Could you check a few things on this model? Use its own coordinates, in mm. A direction names the side the tool comes from. Give positions to 0.01 mm unless a question says otherwise; leave off trailing zeros. Loops run counter-clockwise (first coordinate to the right, second up) from the corner with the lowest first, then second, coordinate; pieces in that order, holes last. Notation, with made-up numbers: (70.25, 31.5) - (115.25, 31.5) arc R21 ccw to (115.25, 57.5) - close; hole circle Ø8 at (5.5, 80.5). An arc over 180 degrees is marked (long way). Write each question's results on one line, items separated by ' | '. Start each with the question number.
(1) Suppose I cut it at A-A (z = 18.5). Please give me the cut outline in (x, y), and give its area (3 significant figures).
(2) Suppose I cut it at D-D (z = -1). Please give me the cut outline in (x, y).
(3) If we mould it in two halves opening along X, with no side actions, what happens to faces 6 (the face through (11.5, 14, -13)), 7 (the face through (0, 0, 0)), 8 (the face through (0, 1.5, 0))? For each: released by +X, released by -X, zero draft, split by the parting line, or undercut.
(4) On a 3-axis mill with a long thin cutter (end or side, diameter ignored), from which of +Z, -Z, +X, -X, +Y, -Y can I reach the whole of each face in a straight line? I mean faces 1 (the face through (2.5, 13.8, -20.5)), 2 (the face through (2, 14, -9)), 3 (the face through (-11, 14, -5.5)), 4 (the face through (-4, 14, -13.5)), 5 (the face through (-11.5, 14, -13)). Say none if no direction works.
(5) Suppose I cut it at C-C (x = -8.5). Please give me the cut outline in (y, z).
(6) For pin 1 (2 mm diameter, centred on y = 19.5, z = -18.5, fed in from -X); pin 2 (1.1 mm diameter, centred on x = 2.5, y = 17, fed in from +Z); pin 3 (7.5 mm diameter, centred on y = 13, z = -7.5, fed in from +X), each with a flat end and sliding along its axis, tell me the tip position at first contact or that it passes through.
(7) Suppose I cut it at B-B (x = -18.5). Please give me the cut outline in (y, z).
(8) I need wall thicknesses on line 1 (Z direction, x = 18.5, y = 0.6); line 2 (X direction, y = 22, z = -12). Which ranges of each line are inside material? Lowest first, please.
from build123d import *

# Parameters (mm, degrees)
SKETCH1_W           = 43
SKETCH1_H           = 43
BOSS_EXTRUDE1_DEPTH = 1.5
SKETCH2_R           = 1.5
CUT_EXTRUDE1_DEPTH  = 2.5
BOSS_EXTRUDE2_DEPTH = 25


with BuildPart() as part:
    # Sketch1 → Boss-Extrude1 (new body)
    with BuildSketch(Plane(origin=(0, 0, 0), x_dir=(1, 0, 0), z_dir=(0, 1, 0))):
        Rectangle(SKETCH1_W, SKETCH1_H)
    extrude(amount=BOSS_EXTRUDE1_DEPTH)

    # Sketch2 → Cut-Extrude1 (cut, through all)
    with BuildSketch(Plane(origin=(0, 1.5, 0), x_dir=(1, 0, 0), z_dir=(0, 1, 0))):
        with Locations((-18.5, 18.5)):
            Circle(SKETCH2_R)
        with Locations((18.5, 18.5)):
            Circle(SKETCH2_R)
        with Locations((18.5, -18.5)):
            Circle(SKETCH2_R)
        with Locations((-18.5, -18.5)):
            Circle(SKETCH2_R)
    extrude(amount=-CUT_EXTRUDE1_DEPTH, mode=Mode.SUBTRACT)

    # Sketch3 → Boss-Extrude2 (add)
    with BuildSketch(Plane(origin=(0, 1.5, 0), x_dir=(1, 0, 0), z_dir=(0, 1, 0))):
        Polygon((-7, 5.5), (-7, 12.5), (-10.5, 12.5), (-10.5, 5.5), (-11.5, 5.5), (-11.5, 20.5), (-10.5, 20.5), (-10.5, 13.5), (-7, 13.5), (-7, 20.5), (-6, 20.5), (-6, 13.5), (-2.5, 13.5), (-2.5, 20.5), (-1.5, 20.5), (-1.5, 13.5), (2, 13.5), (2, 20.5), (3, 20.5), (3, 13.5), (6.5, 13.5), (6.5, 20.5), (7.5, 20.5), (7.5, 13.5), (10.5, 13.5), (10.5, 20.5), (11.5, 20.5), (11.5, 5.5), (10.5, 5.5), (10.5, 12.5), (7.5, 12.5), (7.5, 5.5), (6.5, 5.5), (6.5, 12.5), (3, 12.5), (3, 5.5), (2, 5.5), (2, 12.5), (-1.5, 12.5), (-1.5, 5.5), (-2.5, 5.5), (-2.5, 12.5), (-6, 12.5), (-6, 5.5), align=None)
    extrude(amount=BOSS_EXTRUDE2_DEPTH)


solid = part.part
Output values:
1) outline: (-21.5, 0) - (-20, 0) - (-20, 1.5) - (-21.5, 1.5) - close; (-17, 0) - (17, 0) - (17, 1.5) - (-17, 1.5) - close; (20, 0) - (21.5, 0) - (21.5, 1.5) - (20, 1.5) - close | area: 55.5 mm2
2) outline: (-21.5, 0) - (21.5, 0) - (21.5, 1.5) - (-21.5, 1.5) - close
3) face 6: released by +X | face 7: zero draft | face 8: undercut
4) face 1: -Z, +X, -X, +Y | face 2: +Z, +Y | face 3: +Z, +X, -X, +Y | face 4: -Z, +Y | face 5: +Z, -Z, -X, +Y
5) outline: (0, -21.5) - (1.5, -21.5) - (1.5, -13.5) - (26.5, -13.5) - (26.5, -12.5) - (1.5, -12.5) - (1.5, 21.5) - (0, 21.5) - close
6) pin 1: x = -11.5 | pin 2: z = -5.5 | pin 3: x = 11.5
7) outline: (0, -21.5) - (1.5, -21.5) - (1.5, -20) - (0, -20) - close; (0, -17) - (1.5, -17) - (1.5, 17) - (0, 17) - close; (0, 20) - (1.5, 20) - (1.5, 21.5) - (0, 21.5) - close
8) line 1: -21.5 to -20, -17 to 17, 20 to 21.5 | line 2: -11.5 to -10.5, -7 to -6, -2.5 to -1.5, 2 to 3, 6.5 to 7.5, 10.5 to 11.5
